Autodesk Inventor part; units mm, degrees
ref_plane "工作平面1" through (80, 0, 40) normal (0.0872, 0, 0.9962) x (0, 1, 0)
ref_plane "工作平面2" through (80, 0, 40) normal (0.9962, 0, -0.0872) x (0, 1, 0)
ref_plane "工作平面3" through (40, 0, 40) normal (-1, 0, 0) x (0, 0, 1)
sketch "草圖2" plane through (0, 0, 0) normal (0, 0, 1) x (1, 0, 0)
  line L0 (0, 25) -> (0, 0)
  line L1 (0, 0) -> (10, 0)
  line L2 (10, 0) -> (10, 20)
  line L3 (10, 20) -> (70, 20)
  line L4 (70, 20) -> (70, 0)
  line L5 (70, 0) -> (80, 0)
  line L6 (80, 0) -> (80, 25)
  line L7 (80, 25) -> (0, 25)
  dimension "d11" = 10
  dimension "d12" = 5
  dimension "d14" = 80
  dimension "d17" = 20
extrude "擠出2" add sketch "草圖2" along normal mid plane 80
ref_plane "工作平面1" through (80, 0, 40) normal (0.0872, 0, 0.9962) x (0, 1, 0)
ref_plane "工作平面2" through (80, 0, 40) normal (0.9962, 0, -0.0872) x (0, 1, 0)
ref_plane "工作平面3" through (40, 0, 40) normal (-1, 0, 0) x (0, 0, 1)
equation "\"d11\" = leg_length"
equation "\"d12\" = thickness"
equation "\"d14\" = width"
equation "\"d17\" = height"
equation "\"d15\" = length"
equation "\"width\" = 8 * ratio"
equation "\"height\" = 2 * ratio"
equation "\"length\" = width"
equation "\"leg_length\" = ratio"
equation "\"thickness\" = 0.5 * ratio"
properties part number "bridge_rect_final"
Design review of the part built by this model. Coordinates are the model's own, in mm. A direction names the side the tool comes from. Round coordinates to 2 decimals unless told otherwise and drop trailing zeros. Order: outer loops, then holes, each group sorted by start corner. A loop starts at its lowest first (then second) coordinate and runs counter-clockwise, first axis right, second up.
1) Consider section B-B (z = 6). State the section outline as (x, y) points.
The answers:
outline: (0, 0) - (10, 0) - (10, 20) - (70, 20) - (70, 0) - (80, 0) - (80, 25) - (0, 25) - close
2) Machinability: for faces 1 (the flat face through (75, 0, -1)), 2 (the flat face through (40, 20, -1)), which of the approach directions +Z, -Z, +X, -X, +Y, -Y give a long, thin tool a straight path to every point of the face, cutting with its end or side? Answer none if there is none.
The answers:
face 1: +Z, -Z, +X, -X, -Y
face 2: +Z, -Z, -Y
3) Consider section A-A (y = 9.75). State the section outline as (x, z) points, plus the area to 3 significant figures.
The answers:
outline: (0, -40) - (10, -40) - (10, 40) - (0, 40) - close; (70, -40) - (80, -40) - (80, 40) - (70, 40) - close
area: 1,600 mm2
4) For L1, parallel to X at y = 9.25, z = 5; L2, parallel to Y at x = 52.5, z = -35.5, list the stretches that pass through material, from the lowest coordinate up.
The answers:
L1: x = 0 to 10, 70 to 80
L2: y = 20 to 25
5) Consider section C-C (x = 45). State the section outline as (y, z) points, plus the area to 3 significant figures.
The answers:
outline: (20, -40) - (25, -40) - (25, 40) - (20, 40) - close
area: 400 mm2
6) Clearance check with flat-ended pins moving along their axes: pin 1 Ø1 at (y, z) = (15, 16.5) entering from -X; pin 2 Ø3 at (x, z) = (31, -20.5) entering from -Y. State where each tip first meets the part, or that it passes through.
The answers:
pin 1: stops at x = 0
pin 2: stops at y = 20
